Source: CAD feature listing. Evaluate the final solid. Frame: model axes, mm. Give positions to 0.01 mm unless a question says otherwise; leave off trailing zeros. Loops run counter-clockwise (first coordinate to the right, second up) from the corner with the lowest first, then second, coordinate; pieces in that order, holes last.
```python
from build123d import *

# Parameters (mm, degrees)
ESQUISSE1_W        = 15
ESQUISSE1_H        = 5.05
BOSS_EXTRU_1_DEPTH = 3


with BuildPart() as part:
    # Esquisse1 → Boss.-Extru.1 (new body)
    with BuildSketch(Plane.XY):
        with BuildLine():
            Line((-20, 20), (20, 20))
            ThreePointArc((20, 20), (27.071067812, 17.071067812), (30, 10))
            Line((30, 10), (30, -20))
            Line((30, -20), (-30, -20))
            Line((-30, -20), (-30, 10))
            ThreePointArc((-30, 10), (-27.071067812, 17.071067812), (-20, 20))
        make_face()
        with Locations((15, -14)):
            Rectangle(ESQUISSE1_W, ESQUISSE1_H, mode=Mode.SUBTRACT)
        with Locations((-15, -14)):
            Rectangle(ESQUISSE1_W, ESQUISSE1_H, mode=Mode.SUBTRACT)
    extrude(amount=BOSS_EXTRU_1_DEPTH)


solid = part.part
```
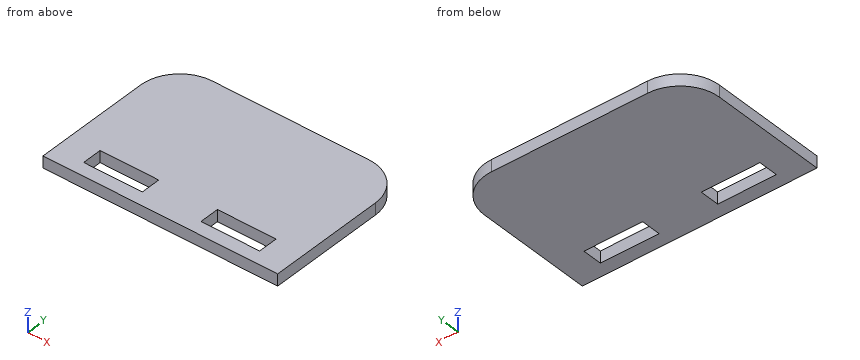
(1) Section C-C, the plane y = 13. Return the cut outline in (x, z).
A:
outline: (-29.54, 0) - (29.54, 0) - (29.54, 3) - (-29.54, 3) - close
(2) Ray query, line 1 along Y through (x, z) = (-11, 0.1) (3 decimals); line 2 along X through (y, z) = (-15.5, 1.9); line 3 along Y through (x, z) = (-22, 0.65) (3 decimals). Return the intervals inside material, ascending.
A:
line 1: y = -20 to -16.525, -11.475 to 20
line 2: x = -30 to -22.5, -7.5 to 7.5, 22.5 to 30
line 3: y = -20 to -16.525, -11.475 to 19.798
(3) Section D-D, the plane x = 24.5. Return the cut outline in (y, z), then the cut area to 3 significant figures.
A:
outline: (-20, 0) - (18.93, 0) - (18.93, 3) - (-20, 3) - close
area: 117 mm2
(4) First-contact query: pin 1 (1.5 mm diameter, centred on x = -22.5, z = 2, fed in from +Y). Flat tip, straight axial feed; report the tip coordinate or a pass-through.
A:
pin 1: stops at y = 19.85
(5) Section A-A, the plane x = -18.5. Return the cut outline in (y, z) (3 decimals).
A:
outline: (-20, 0) - (-16.525, 0) - (-16.525, 3) - (-20, 3) - close; (-11.475, 0) - (20, 0) - (20, 3) - (-11.475, 3) - close
(6) Section B-B, the plane z = 0.9. Return the cut outline in (x, y) (3 decimals), then the cut area to 3 significant figures.
A:
outline: (-30, -20) - (30, -20) - (30, 10) arc R10 ccw to (20, 20) - (-20, 20) arc R10 ccw to (-30, 10) - close; hole (-22.5, -16.525) - (-7.5, -16.525) - (-7.5, -11.475) - (-22.5, -11.475) - close; hole (7.5, -16.525) - (22.5, -16.525) - (22.5, -11.475) - (7.5, -11.475) - close
area: 2,210 mm2
